```python
from build123d import *

# Parameters (mm, degrees)
F0_R           = 35
F1_DEPTH       = 16
F2_R           = 20.5
F3_DEPTH       = 2.5
F4_R           = 4
F5_DEPTH       = 8
F6_D           = 5.5
F6_CSINK_D     = 11.2
F6_CSINK_ANGLE = 90
F7_R           = 2.5
F8_DEPTH       = 5
F9_SIZE        = 1


with BuildPart() as f1:
    # F0 (on Top) → F1 (new body)
    with BuildSketch(Plane.XY):
        Circle(F0_R)
    extrude(amount=F1_DEPTH)

    # F2 (on face) → F3 (cut)
    with BuildSketch(Plane(origin=(0, 0, 0), x_dir=(1, 0, 0), z_dir=(0, 0, -1))):
        Circle(F2_R)
    extrude(amount=-F3_DEPTH, mode=Mode.SUBTRACT)

    # F4 (on face) → F5 (cut)
    with BuildSketch(Plane.XY.offset(16)):
        with Locations((0, 27)):
            Circle(F4_R)
        with Locations((19.091883092, -19.091883092)):
            Circle(F4_R)
        with Locations((-19.091883092, -19.091883092)):
            Circle(F4_R)
    extrude(amount=-F5_DEPTH, mode=Mode.SUBTRACT)

    # F6 (through all)
    with Locations(Plane.XY.offset(16)):
        with Locations((-11.1369318037, 11.1369318037), (11.1369318037, 11.1369318037), (0, -15.75)):
            CounterSinkHole(F6_D / 2, F6_CSINK_D / 2, counter_sink_angle=F6_CSINK_ANGLE)

    # F7 (on face) → F8 (cut)
    with BuildSketch(Plane(origin=(0, 0, 2.5), x_dir=(1, 0, 0), z_dir=(0, 0, -1))):
        with Locations((0, -15.75)):
            Circle(F7_R)
    extrude(amount=-F8_DEPTH, mode=Mode.SUBTRACT)

    # F9
    f9_edges = [f1.edges().sort_by_distance(p)[0] for p in [
        (-20.5, 0, 0),
        (-35, 0, 0),
        (-35, 0, 16),
        (-23.091883, -19.091883, 16),
        (-4, 27, 16),
        (15.091883, -19.091883, 16),
    ]]
    chamfer(f9_edges, length=F9_SIZE)


solid = f1.part
```
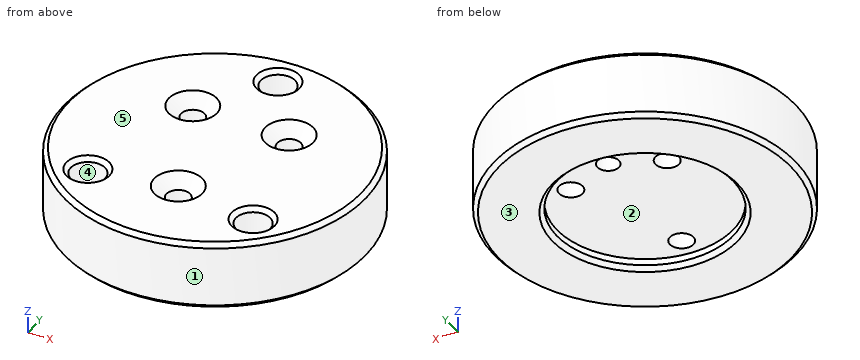
Verification items for the finished model (mm, model axes). Face numbers are marked on the shaded views. A direction names the side the tool comes from. Coordinates: 2 decimals unless noted, no trailing zeros. Write each loop counter-clockwise with the first axis right and the second up, starting at its lowest first coordinate (ties: lowest second). Pieces come first, ordered by that corner, then holes. Notation, with made-up numbers: M 69.5,76.25 L 126.5,76.25 A21 ccw 126.5,107.25 Z; hole C 55,47.5 d5. An arc over 180 degrees is marked long. One line per item, written item: value.
Item 1: Access from +Z, -Z, +X, -X, +Y, -Y to the whole of each face (thin tool, end or side, straight path). Record for the marked faces 4 and 5.
Check sheet entries:
face 4: +Z
face 5: +Z, +X, -X, +Y, -Y
Item 2: Mould release check, pull along X, two halves, no side actions. Record for the marked faces 1, 2 and 3: pulls with the +X half, pulls with the -X half, needs draft (parallel to the pull), parting line crosses it, or undercut.
Check sheet entries:
face 1: parting line crosses it
face 2: undercut
face 3: needs draft
Item 3: Section check B-B, the plane y = 0. Record the boundary of the cut face in (x, z), plus the area to 3 significant figures.
Check sheet entries:
outline: M -35,1 L -34,0 L -21.5,0 L -20.5,1 L -20.5,2.5 L 20.5,2.5 L 20.5,1 L 21.5,0 L 34,0 L 35,1 L 35,15 L 34,16 L -34,16 L -35,15 Z
area: 1,010 mm^2
Item 4: Gauge pin test, flat ends, axial feed: pin 1 Ø10.5 at (x, y) = (-19.09, -19.09) entering from +Z; pin 2 Ø4 at (y, z) = (15, 9) entering from -X; pin 3 Ø3 at (x, y) = (-15.5, 2.5) entering from -Z; pin 4 Ø5 at (x, y) = (0, 27) entering from +Z. Record the tip position at first contact, or that the pin passes through.
Check sheet entries:
pin 1: stops at z = 16
pin 2: stops at x = -32.5
pin 3: stops at z = 2.5
pin 4: stops at z = 8
Item 5: Scan lines: line 1 along Y through (x, z) = (0, 5.35); line 2 along Y through (x, z) = (-2, 6); line 3 along X through (y, z) = (-20, 9). Record each from-to range of solid material in increasing order.
Check sheet entries:
line 1: y = -35 to -18.5, -13 to 13.25, 18.25 to 35
line 2: y = -34.94 to -17.64, -13.86 to 14.25, 17.25 to 34.94
line 3: x = -28.72 to -22.99, -15.2 to 15.2, 22.99 to 28.72
